```python
from build123d import *

# Parameters (mm, degrees)
SKETCH1_W           = 30.48
SKETCH1_H           = 30.48
BOSS_EXTRUDE1_DEPTH = 3.175
CUT_EXTRUDE1_REACH  = 8.35
SKETCH2_R           = 3.175


with BuildPart() as part:
    # Sketch1 → Boss-Extrude1 (new body, symmetric)
    with BuildSketch(Plane(origin=(0, 0, 0), x_dir=(1, 0, 0), z_dir=(0, 1, 0))):
        Rectangle(SKETCH1_W, SKETCH1_H)
    extrude(amount=BOSS_EXTRUDE1_DEPTH, both=True)

    # Sketch2 → Cut-Extrude1 (cut, up to next)
    with BuildSketch(Plane(origin=(0, 3.175, 0), x_dir=(1, 0, 0), z_dir=(0, 1, 0)), mode=Mode.PRIVATE) as cut_extrude1_sk1:
        with Locations((9.525, 0)):
            Circle(SKETCH2_R)
    cut_extrude1_tool1 = extrude(cut_extrude1_sk1.sketch, amount=-CUT_EXTRUDE1_REACH, mode=Mode.PRIVATE) & part.part
    add(cut_extrude1_tool1.solids().sort_by_distance((9.525, 3.175, 0))[0], mode=Mode.SUBTRACT)
    # Sketch2 → Cut-Extrude1 (cut, up to next)
    with BuildSketch(Plane(origin=(0, 3.175, 0), x_dir=(1, 0, 0), z_dir=(0, 1, 0)), mode=Mode.PRIVATE) as cut_extrude1_sk2:
        with Locations((-8.255, -7.62)):
            Circle(SKETCH2_R)
    cut_extrude1_tool2 = extrude(cut_extrude1_sk2.sketch, amount=-CUT_EXTRUDE1_REACH, mode=Mode.PRIVATE) & part.part
    add(cut_extrude1_tool2.solids().sort_by_distance((-8.255, 3.175, 7.62))[0], mode=Mode.SUBTRACT)
    # Sketch2 → Cut-Extrude1 (cut, up to next)
    with BuildSketch(Plane(origin=(0, 3.175, 0), x_dir=(1, 0, 0), z_dir=(0, 1, 0)), mode=Mode.PRIVATE) as cut_extrude1_sk3:
        with Locations((-8.255, 7.62)):
            Circle(SKETCH2_R)
    cut_extrude1_tool3 = extrude(cut_extrude1_sk3.sketch, amount=-CUT_EXTRUDE1_REACH, mode=Mode.PRIVATE) & part.part
    add(cut_extrude1_tool3.solids().sort_by_distance((-8.255, 3.175, -7.62))[0], mode=Mode.SUBTRACT)


solid = part.part
```
Design review of the part built by this model. Coordinates are the model's own, in mm. Coordinates: 2 decimals unless noted, no trailing zeros. Order: outer loops, then holes, each group sorted by start corner. A loop starts at its lowest first (then second) coordinate and runs counter-clockwise, first axis right, second up. Notation, with made-up numbers: M 75,-30.5 L 98,-30.5 A13 cw 98,-24.5 Z; hole C 87,73 d9. An arc over 180 degrees is marked long. Answer as a JSON object with one key per item and string values. Group by question number.
1) Wall thickness on L1, parallel to Z at x = -8.5, y = -0.5; L2, parallel to X at y = 2, z = 0; L3, parallel to Z at x = -6.5, y = -2: over which ranges is each line inside the solid? List them lowest first.
2) Add section C-C, the plane x = -6.5. Write out the cut boundary in (y, z) (3 decimals).
3) Add section A-A, the plane z = 0. Write out the cut boundary in (x, y) (3 decimals), then the cut area to 3 significant figures.
4) Add section D-D, the plane z = -10. Write out the cut boundary in (x, y) (3 decimals), then the cut area to 3 significant figures.
5) Mouldability with a two-part tool opening along X and no side actions: class faces 1 (the cylindrical face through (12.458, 0.044, 1.216)), 2 (the flat face through (0, 0, 15.24)), 3 (the flat face through (-15.24, 0, 0)) as pulls with the +X half, pulls with the -X half, needs draft (parallel to the pull), parting line crosses it, or undercut.
6) Add section B-B, the plane y = -0.5. Write out the cut boundary in (x, z) (3 decimals).
Computed values:
{
 "1": {"L1": "z = -15.24 to -10.79, -4.45 to 4.45, 10.79 to 15.24", "L2": "x = -15.24 to 6.35, 12.7 to 15.24", "L3": "z = -15.24 to -10.27, -4.97 to 4.97, 10.27 to 15.24"},
 "2": {"outline": "M -3.175,-15.24 L 3.175,-15.24 L 3.175,-10.266 L -3.175,-10.266 Z; M -3.175,-4.974 L 3.175,-4.974 L 3.175,4.974 L -3.175,4.974 Z; M -3.175,10.266 L 3.175,10.266 L 3.175,15.24 L -3.175,15.24 Z"},
 "3": {"outline": "M -15.24,-3.175 L 6.35,-3.175 L 6.35,3.175 L -15.24,3.175 Z; M 12.7,-3.175 L 15.24,-3.175 L 15.24,3.175 L 12.7,3.175 Z", "area": "153 mm^2"},
 "4": {"outline": "M -15.24,-3.175 L -10.356,-3.175 L -10.356,3.175 L -15.24,3.175 Z; M -6.154,-3.175 L 15.24,-3.175 L 15.24,3.175 L -6.154,3.175 Z", "area": "167 mm^2"},
 "5": {"face 1": "undercut", "face 2": "needs draft", "face 3": "pulls with the -X half"},
 "6": {"outline": "M -15.24,-15.24 L 15.24,-15.24 L 15.24,15.24 L -15.24,15.24 Z; hole C -8.255,-7.62 d6.35; hole C -8.255,7.62 d6.35; hole C 9.525,0 d6.35"}
}
